Autodesk Inventor part; units mm, degrees
ref_plane "Work Plane1" through (3.5, 0, 0) normal (0, 0, 1) x (1, 0, 0)
ref_plane "YZ Plane" through (0, 0, 0) normal (1, 0, 0) x (0, 1, 0)
ref_plane "XZ Plane" through (0, 0, 0) normal (0, 1, 0) x (-1, 0, 0)
sketch "Sketch1" plane through (0, 0, 0) normal (0, 0, 1) x (1, 0, 0)
  line L0 (0, 9.906) -> (0, 4.7625)
  line L1 (13.335, 4.7625) -> (88.9, 4.7625)
  line L2 (88.9, 4.7625) -> (88.9, 0)
  line L3 (88.9, 0) -> (-1.6002, 0)
  line L4 (0, -1.9812) -> (0, 11.8872)
  line L5 (-19.7002, 0) -> (107, 0)
  line L6 (-1.6002, 0) -> (-1.6002, 9.906)
  line L7 (-1.6002, 9.906) -> (0, 9.906)
  line L8 (13.335, 4.7625) -> (12.5412, 4.7625)
  line L9 (12.5412, 4.7625) -> (0, 4.7625)
  dimension "d0" = 88.9
  dimension "d1" = 75.565
  dimension "d2" = 9.525
  dimension "d8" = 1.6002
  dimension "d9" = 19.812
  dimension "d15" = 9.525
  dimension "d16" = 0.7937
revolve "Body" add sketch "Sketch1" angle 360 about axis through (88.9, 0, 0) along (-1, 0, 0)
sketch "Sketch2" plane through (0, 0, 0) normal (1, 0, 0) x (0, 0, -1)
  circle A0 centre (0, 0) radius 9.906
  line L0 (0, 8.2416) -> (7.1374, 4.1208)
  line L1 (7.1374, 4.1208) -> (7.1374, -4.1208)
  line L2 (7.1374, -4.1208) -> (0, -8.2416)
  line L3 (0, -8.2416) -> (-7.1374, -4.1208)
  line L4 (-7.1374, -4.1208) -> (-7.1374, 4.1208)
  line L5 (-7.1374, 4.1208) -> (0, 8.2416)
  circle A1 centre (0, 0) radius 9.906
  dimension "d10" = 14.2748
extrude "Head" add sketch "Sketch2" against normal blind 7.493 contours L0 L1 L2 L3 L4 L5
sketch "Sketch3" plane through (0, 0, 0) normal (0, 0, 1) x (1, 0, 0)
  line L0 (-7.493, 7.1374) -> (-7.493, 8.2416)
  line L1 (-7.493, 8.2416) -> (-6.8555, 8.2416)
  line L2 (-6.8555, 8.2416) -> (-7.493, 7.1374)
  line L3 (-2.8347, 8.2416) -> (-7.493, 8.2416)
  line L4 (-7.493, 8.2416) -> (-7.493, 5.9322)
  line L5 (-1.6002, 8.2416) -> (-7.493, 8.2416)
  line L6 (-7.493, 8.2416) -> (-7.493, 4.1208)
  line L7 (-8.6716, 0) -> (-0.4216, 0)
  dimension "d5" = 30
  dimension "d18" = 14.2748
revolve "Chamfer1" cut sketch "Sketch3" angle 360 about axis through (-10, 0, 0) along (1, 0, 0)
thread "Thread"
chamfer "Chamfer2" distance 0.7938 distance2 0.7938 1 edges at (88.9, -4.7625, 0) measured on face at (88.9, 1.1883, -1.0527)
ref_plane "Work Plane1" through (3.5, 0, 0) normal (0, 0, 1) x (1, 0, 0)
equation "\"d0\" = NLG"
equation "\"d1\" = GEL"
equation "\"d2\" = GD"
equation "\"d8\" = PHH"
equation "\"d9\" = LADI"
equation "\"d15\" = BDM"
equation "\"d16\" = GAL"
equation "\"d10\" = SW"
equation "\"d3\" = KOH"
equation "\"d13\" = GEL"
equation "\"d6\" = -0.5 * SPD + 0.5 * GD"
equation "\"d7\" = -0.5 * SPD + 0.5 * GD"
equation "\"d5\" = ANG1"
equation "\"d18\" = SW0"
equation "\"NLG\" = 88.9"
equation "\"GD\" = NND"
equation "\"BDM\" = NND"
equation "\"KOH\" = 7.493"
equation "\"GEL\" = 75.565"
equation "\"LADI\" = 19.812"
equation "\"SW\" = 14.2748"
equation "\"PHH\" = 1.6002"
equation "\"SW0\" = 14.2748"
equation "\"SPD\" = GD1"
equation "\"ANG1\" = 30deg"
equation "\"GAL\" = 0.79375"
equation "\"GUL\" = GAL"
equation "\"GD1\" = 7.9375"
equation "\"THREADDIA\" = 9.525"
equation "\"SDH\" = SW"
equation "\"TOA\" = 30deg"
equation "\"RR\" = 0.09525"
equation "\"NND\" = 9.525"
equation "\"SD\" = 0"
equation "\"SD2\" = NND"
equation "\"E0\" = 16.48739"
properties part number "ANSI B18.6.3 - 3/8-16 UNC x 3.5, PHWHMSI" material "Steel, Mild"
Can you work these out from the model? Positions are in its coordinate system, mm. A direction names the side the tool comes from. Coordinates: 2 decimals unless noted, no trailing zeros. Write each loop counter-clockwise with the first axis right and the second up, starting at its lowest first coordinate (ties: lowest second). Pieces come first, ordered by that corner, then holes. Notation, with made-up numbers: (-14, -30) -> (37, -30) arc R24 ccw to (37, -6) -> close; hole circle Ø3 at (-2.75, 25.25). An arc over 180 degrees is marked (long way). Write each question's results on one line, items separated by ' | '. Start each with the question number.
Q1. Imagine slicing it at B-B (z = 8.75). Write out the boundary of the cut face in (x, y), then the cut area to 3 significant figures.
Q2. If I drill on probe 1 along X at (y, z) = (-4, 5); probe 2 along X at (y, z) = (-3.75, -7.75); probe 3 along Y at (x, z) = (16, 4), over which ranges is the centre line in solid material (lowest first)?
Q3. I'm going to push flat-ended pins straight in: pin 1 (8 mm diameter, centred on x = 65, y = 4.5, fed in from +Z); pin 2 (10 mm diameter, centred on x = 61.5, z = 3, fed in from +Y); pin 3 (1 mm diameter, centred on x = 8.5, z = 5.5, fed in from -Y); pin 4 (1.8 mm diameter, centred on x = -5, y = 1.5, fed in from -Z). Where does each tip first touch, or does it pass through?
Q4. On a 3-axis mill with a long thin cutter (end or side, diameter ignored), from which of +Z, -Z, +X, -X, +Y, -Y can I reach the whole of each face in a straight line? I mean faces 1 (the face through (43.44, -3.78, 2.9)), 2 (the face through (-4.51, 6.21, -3.52)), 3 (the face through (-5, 0, -7.137)), 4 (the face through (-4.51, -6.21, 3.52)). Say none if no direction works.
Q5. Imagine slicing it at A-A (x = 17.5). Write out the boundary of the cut face in (y, z) (1 decimal).
Taken from the geometry:
1) outline: (-1.6, -4.64) -> (0, -4.64) -> (0, 4.64) -> (-1.6, 4.64) -> close | area: 14.9 mm^2
2) probe 1: x = -7.49 to 0 | probe 2: x = -1.6 to 0 | probe 3: y = -2.58 to 2.58
3) pin 1: stops at z = 4.74 | pin 2: stops at y = 4.76 | pin 3: passes through | pin 4: stops at z = -7.14
4) face 1: +X | face 2: -Z, -X, +Y | face 3: -Z, -X, +Y, -Y | face 4: +Z, -X, -Y
5) outline: circle Ø9.5 at (0, 0)
